Could you check a few things on this model? Use its own coordinates, in mm. Face numbers are marked on the shaded views. A direction names the side the tool comes from. Coordinates: 2 decimals unless noted, no trailing zeros. Order: outer loops, then holes, each group sorted by start corner. A loop starts at its lowest first (then second) coordinate and runs counter-clockwise, first axis right, second up. Notation, with made-up numbers: (80, -1.5) - (91, -1.5) arc R11 ccw to (91, 19.5) - close; hole circle Ø3 at (81, 13.25). An arc over 180 degrees is marked (long way). One line per item, written item: value.
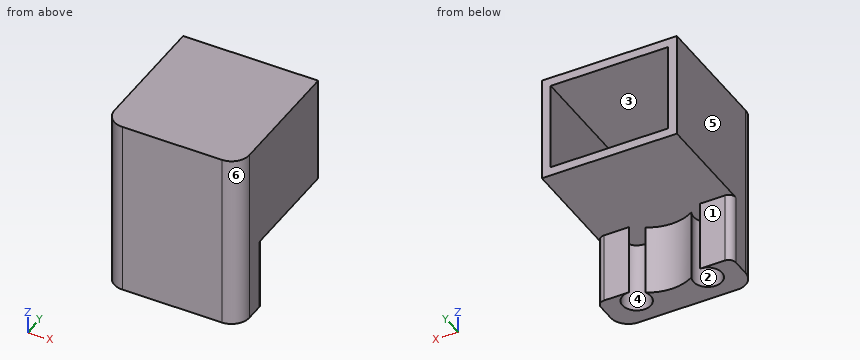
from build123d import *

# Parameters (mm, degrees)
BOSS_EXTRUDE1_DEPTH = 10
SKETCH2_W           = 38
SKETCH2_H           = 40
BOSS_EXTRUDE2_DEPTH = 30
FILLET1_R           = 5
FILLET2_R           = 2
SKETCH4_W           = 33
SKETCH4_H           = 25
CUT_EXTRUDE1_DEPTH  = 35


with BuildPart() as part:
    # Sketch1 → Boss-Extrude1 (new, symmetric)
    with BuildSketch(Plane.XY):
        with BuildLine():
            Line((-10, -9.124404748), (-19, -9.124404748))
            Line((-19, -9.124404748), (-19, -21.124404748))
            Line((-19, -21.124404748), (19, -21.124404748))
            Line((19, -21.124404748), (19, -9.124404748))
            Line((19, -9.124404748), (10, -9.124404748))
            ThreePointArc((10, -9.124404748), (12.023420987, -16.574878268), (6.509119733, -11.171520993))
            ThreePointArc((6.509119733, -11.171520993), (0, -13), (-6.509119733, -11.171520993))
            ThreePointArc((-6.509119733, -11.171520993), (-12.023420987, -16.574878268), (-10, -9.124404748))
        make_face()
    extrude(amount=BOSS_EXTRUDE1_DEPTH, both=True)

    # Sketch2 → Boss-Extrude2 (add)
    with BuildSketch(Plane.XY.offset(10)):
        with Locations((0, -1.124404748)):
            Rectangle(SKETCH2_W, SKETCH2_H)
    extrude(amount=BOSS_EXTRUDE2_DEPTH)

    # Fillet1
    fillet1_edges = [part.edges().sort_by_distance(p)[0] for p in [
        (19, -21.124404748, 15),
        (-19, -21.124404748, 15),
    ]]
    fillet(fillet1_edges, radius=FILLET1_R)

    # Fillet2
    fillet2_edges = [part.edges().sort_by_distance(p)[0] for p in [
        (19, -9.124404748, 0),
        (-19, -9.124404748, 0),
    ]]
    fillet(fillet2_edges, radius=FILLET2_R)

    # Sketch4 → Cut-Extrude1 (cut)
    with BuildSketch(Plane(origin=(0, 18.875595252, 0), x_dir=(1, 0, 0), z_dir=(0, 1, 0))):
        with Locations((0, -25)):
            Rectangle(SKETCH4_W, SKETCH4_H)
    extrude(amount=-CUT_EXTRUDE1_DEPTH, mode=Mode.SUBTRACT)


solid = part.part
Item 1: I'm going to push flat-ended pins straight in: pin 1 Ø2 at (x, z) = (-14.5, -2) entering from +Y; pin 2 Ø10 at (x, y) = (-0.5, 5.5) entering from -Z; pin 3 Ø4 at (x, z) = (-7, 35) entering from +Y. Where does each tip first touch, or does it pass through?
Conclusion:
pin 1: y = -9.12
pin 2: z = 10
pin 3: y = -16.12
Item 2: Thinking about a two-plate mould opening in Y: for the marked faces 4, 5 and 6, which applies, pulls with the +Y half, pulls with the -Y half, needs draft (parallel to the pull), parting line crosses it, or undercut?
Conclusion:
face 4: undercut
face 5: needs draft
face 6: pulls with the -Y half
Item 3: I want a section at D-D on z = 36. Please give me the cut outline in (x, y), then the cut area to 3 significant figures.
Conclusion:
outline: (-19, -16.12) arc R5 ccw to (-14, -21.12) - (14, -21.12) arc R5 ccw to (19, -16.12) - (19, 18.88) - (16.5, 18.88) - (16.5, -16.12) - (-16.5, -16.12) - (-16.5, 18.88) - (-19, 18.88) - close
area: 354 mm²
Item 4: I want a section at C-C on x = -11. Please give me the cut outline in (y, z), then the cut area to 3 significant figures.
Conclusion:
outline: (-21.12, -10) - (-17, -10) - (-17, 10) - (-9.25, 10) - (-9.25, -10) - (-9.12, -10) - (-9.12, 10) - (18.88, 10) - (18.88, 12.5) - (-16.12, 12.5) - (-16.12, 37.5) - (18.88, 37.5) - (18.88, 40) - (-21.12, 40) - close
area: 410 mm²
Item 5: For the marked faces 1, 2 and 3, which set-ups out of +Z, -Z, +X, -X, +Y, -Y let a thin tool reach every point of the face, with its end or its side?
Conclusion:
face 1: -Z, +X, -X, +Y
face 2: -Z
face 3: +Y
Item 6: I want a section at A-A on y = 4. Please give me the cut outline in (x, z), then the cut area to 3 significant figures.
Conclusion:
outline: (-19, 10) - (19, 10) - (19, 40) - (-19, 40) - close; hole (-16.5, 12.5) - (16.5, 12.5) - (16.5, 37.5) - (-16.5, 37.5) - close
area: 315 mm²
Item 7: If I drill on probe 1 along Z at (x, y) = (9, -3.5); probe 2 along X at (y, z) = (11, 19.5); probe 3 along Z at (x, y) = (-15.5, -15.5), over which ranges is the centre line in solid material (lowest first)?
Conclusion:
probe 1: 10 to 12.5, 37.5 to 40
probe 2: -19 to -16.5, 16.5 to 19
probe 3: -10 to 12.5, 37.5 to 40
Item 8: I want a section at B-B on z = -4.5. Please give me the cut outline in (x, y).
Conclusion:
outline: (-19, -16.12) arc R5 ccw to (-14, -21.12) - (14, -21.12) arc R5 ccw to (19, -16.12) - (19, -11.12) arc R2 ccw to (17, -9.12) - (10, -9.12) arc R4 cw (long way) to (6.51, -11.17) arc R12.5 cw to (-6.51, -11.17) arc R4 cw (long way) to (-10, -9.12) - (-17, -9.12) arc R2 ccw to (-19, -11.12) - close
